Geometry check sheet. Reference: the model listing, model coordinates, mm. A direction names the side the tool comes from. Give positions to 0.01 mm unless a question says otherwise; leave off trailing zeros. Write each loop counter-clockwise with the first axis right and the second up, starting at its lowest first coordinate (ties: lowest second). Pieces come first, ordered by that corner, then holes.
(1) Mould release check, pull along Z, two halves, no side actions. Record for faces 1 (the cylindrical face through (-137.744, 11.732, -4.864)), 2 (the flat face through (-2.54, 0, -9)), 3 (the flat face through (-25.4, 0, 0)): +Z half, -Z half, draft (parallel to the pull), parting line (faces both ways), or undercut.
(2) Cross-section at C-C (x = -111.5). Record the boundary of the cut face in (y, z).
(3) Depth check by flat-ended pin: P1, Ø3, axis at x = -1, y = 9.5, coming from the +Z side; P2, Ø1.3, axis at x = -1.5, z = 10, coming from the -Y side; P3, Ø1.5, axis at x = -53.5, z = 1.5, coming from the +Y side. Enter the tip coordinate at first touch or a pass-through.
(4) Cross-section at A-A (z = 0). Record the boundary of the cut face in (x, y), and give its area (3 significant figures).
(5) Tool access check on faces 4 (the flat face through (-2.54, 9, 0)), 5 (the flat face through (0, 6, 6)), 6 (the flat face through (-2.54, 0, 9)). Record the directions out of +Z, -Z, +X, -X, +Y, -Y that give a thin tool (end or side, any length) a straight path to the whole face; none if there is none.
(6) Thickness scan on line 1 along Z through (x, y) = (-15, 0); line 2 along Y through (x, z) = (-243, -2.75); line 3 along X through (y, z) = (0.25, 10.5). Record the ranges inside material, lowest first.
```python
from build123d import *

# Parameters (mm, degrees)
F0_R     = 12.7
F1_DEPTH = 279.4
F2_R     = 6.35
F3_DEPTH = 25.4
F5_DEPTH = 2.54


with BuildPart() as f1:
    # F0 (on Right) → F1 (new body)
    with BuildSketch(Plane.YZ):
        Circle(F0_R)
    extrude(amount=-F1_DEPTH)

    # F2 (on face) → F3 (cut)
    with BuildSketch(Plane.YZ):
        Circle(F2_R)
    extrude(amount=-F3_DEPTH, mode=Mode.SUBTRACT)

    # F4 (on Right) → F5 (cut)
    with BuildSketch(Plane.YZ):
        with BuildLine():
            ThreePointArc((2.54, -5.819871), (0, -6.35), (-2.54, -5.819871))
            Line((-2.54, -5.819871), (-2.54, -12.443408))
            ThreePointArc((-2.54, -12.443408), (0, -12.7), (2.54, -12.443408))
            Line((2.54, -12.443408), (2.54, -5.819871))
        make_face()
        with BuildLine():
            ThreePointArc((-5.819871, -2.54), (-6.35, 0), (-5.819871, 2.54))
            Line((-5.819871, 2.54), (-12.443408, 2.54))
            ThreePointArc((-12.443408, 2.54), (-12.7, 0), (-12.443408, -2.54))
            Line((-12.443408, -2.54), (-5.819871, -2.54))
        make_face()
        with BuildLine():
            ThreePointArc((2.54, 12.443408), (0, 12.7), (-2.54, 12.443408))
            Line((-2.54, 12.443408), (-2.54, 5.819871))
            ThreePointArc((-2.54, 5.819871), (-4.490128, 4.490128), (-5.819871, 2.54))
            ThreePointArc((-5.819871, 2.54), (-6.35, 0), (-5.819871, -2.54))
            ThreePointArc((-5.819871, -2.54), (-4.490128, -4.490128), (-2.54, -5.819871))
            ThreePointArc((-2.54, -5.819871), (0, -6.35), (2.54, -5.819871))
            ThreePointArc((2.54, -5.819871), (4.490128, -4.490128), (5.819871, -2.54))
            ThreePointArc((5.819871, -2.54), (6.35, 0), (5.819871, 2.54))
            ThreePointArc((5.819871, 2.54), (4.490128, 4.490128), (2.54, 5.819871))
            Line((2.54, 5.819871), (2.54, 12.443408))
        make_face()
        with BuildLine():
            Line((12.443408, 2.54), (5.819871, 2.54))
            ThreePointArc((5.819871, 2.54), (6.35, 0), (5.819871, -2.54))
            Line((5.819871, -2.54), (12.443408, -2.54))
            ThreePointArc((12.443408, -2.54), (12.7, 0), (12.443408, 2.54))
        make_face()
    extrude(amount=-F5_DEPTH, mode=Mode.SUBTRACT)


solid = f1.part
```
Reply:
1. face 1: parting line
1. face 2: draft
1. face 3: undercut
2. outline: circle Ø25.4 at (0, 0)
3. P1: stops at z = 9.86
3. P2: stops at y = -8.59
3. P3: stops at y = 12.68
4. outline: (-279.4, -12.7) - (-2.54, -12.7) - (-2.54, -6.35) - (-25.4, -6.35) - (-25.4, 6.35) - (-2.54, 6.35) - (-2.54, 12.7) - (-279.4, 12.7) - close
4. area: 6,740 mm2
5. face 4: +X, +Y, -Y
5. face 5: +Z, -Z, +X, +Y, -Y
5. face 6: +Z, -Z, +X
6. line 1: z = -12.7 to -6.35, 6.35 to 12.7
6. line 2: y = -12.4 to 12.4
6. line 3: x = -279.4 to -2.54
